Source: CAD feature listing. Evaluate the final solid. Frame: model axes, mm. A direction names the side the tool comes from. Round coordinates to 2 decimals unless told otherwise and drop trailing zeros. Order: outer loops, then holes, each group sorted by start corner. A loop starts at its lowest first (then second) coordinate and runs counter-clockwise, first axis right, second up. Notation, with made-up numbers: (76, 84) -> (113, 84) arc R23 ccw to (113, 99) -> close; hole circle Ø4 at (-27, 69.5). An arc over 180 degrees is marked (long way). Answer as CSV lines item,"result". Start each with the question number.
(1) Contact query for a flat-ended pin moving along its axis: P1, Ø4, axis at x = 2, z = 37, coming from the +Y side. Output: stop coordinate, or through.
(2) Section query B-B (z = 27.5). Output: boundary loops of the cut face in (x, y).
(3) Section query A-A (y = 2.95). Output: boundary loops of the cut face in (x, z), plus the area to 3 significant figures.
(4) Set-up query: faces 1 (the cylindrical face through (-0.2, 0.56, -38.91)), 2 (the flat face through (-0.09, 1.1, 35.77)). Return all of +Z, -Z, +X, -X, +Y, -Y with unobstructed straight access to the full face (end or side cutting, diameter ignored); none if empty.
(5) Pull-direction query (Z, two-part tool) for faces 3 (the flat face through (11.25, 2, 1)), 4 (the cylindrical face through (-0.2, 0.56, -11.26)), 5 (the cylindrical face through (10.537, 2.021, 41.748)); classes: +Z half, -Z half, draft (parallel to the pull), parting line (faces both ways), or undercut.
(6) Section query C-C (x = 0). Count the separate pieces of the cut face and the enclosed holes in it, plus the area to 3 significant figures.
(7) Line query: line 1 along Z through (x, y) = (-3, 3.9); line 2 along X through (y, z) = (3, -7.5); line 3 along Y through (x, z) = (-3.5, 11). Output: solid intervals per line, ascending. Write a range as from..to.
Autodesk Inventor part; units mm, degrees
ref_plane "YZ Plane" through (0, 0, 0) normal (1, 0, 0) x (0, 1, 0)
ref_plane "XZ Plane" through (0, 0, 0) normal (0, 1, 0) x (-1, 0, 0)
ref_plane "XY Plane" through (0, 0, 0) normal (0, 0, 1) x (1, 0, 0)
sketch "Szkic1" plane through (0, 0, 0) normal (0, 1, 0) x (-1, 0, 0)
  line L0 (8.75, 42.5) -> (-8.75, 42.5)
  line L1 (-11.25, 40) -> (-11.25, -40)
  line L2 (-8.75, -42.5) -> (8.75, -42.5)
  line L3 (11.25, -40) -> (11.25, 40)
  line L4 (-11.25, 42.5) -> (11.25, -42.5)
  line L5 (-11.25, -42.5) -> (11.25, 42.5)
  arc A0 (11.25, 40) -> (8.75, 42.5) centre (8.75, 40) ccw
  arc A1 (-8.75, 42.5) -> (-11.25, 40) centre (-8.75, 40) ccw
  arc A2 (-11.25, -40) -> (-8.75, -42.5) centre (-8.75, -40) ccw
  arc A3 (8.75, -42.5) -> (11.25, -40) centre (8.75, -40) ccw
  point P0 (0, 0)
  point P1 (0, 0)
  dimension "d0" = 22.5
  dimension "d1" = 85
  dimension "d2" = 2.5
extrude "Wyciągnięcie proste1" add sketch "Szkic1" along normal blind 4.1
sketch "Szkic2" plane through (0, 4.1, 0) normal (0, 1, 0) x (1, 0, 0)
  line L0 (-6.3, -35) -> (6.3, -35)
  line L1 (6.3, -35) -> (6.3, -12.2)
  line L2 (6.3, -12.2) -> (-6.3, -12.2)
  line L3 (-6.3, -12.2) -> (-6.3, -35)
  line L4 (-8.75, -42.5) -> (8.75, -42.5)
  line L5 (11.25, -40) -> (11.25, 40)
  line L6 (-6.3, 12.2) -> (6.3, 12.2)
  line L7 (6.3, 12.2) -> (6.3, 35)
  line L8 (6.3, 35) -> (-6.3, 35)
  line L9 (-6.3, 35) -> (-6.3, 12.2)
  line L10 (-15.75, 0) -> (15.75, 0)
  point P0 (0, 0)
  point P1 (0, -35)
  dimension "d5" = 12.6
  dimension "d6" = 22.8
  dimension "d7" = 7.5
  dimension "d8" = 11.25
extrude "Wyciągnięcie proste2" cut sketch "Szkic2" against normal blind 4.1
sketch "Szkic4" plane through (0, 4.1, 0) normal (0, 1, 0) x (1, 0, 0)
  line L0 (-6.3, -39.85) -> (6.3, -39.85)
  line L1 (6.3, -39.85) -> (6.3, -7.35)
  line L2 (6.3, -7.35) -> (-6.3, -7.35)
  line L3 (-6.3, -7.35) -> (-6.3, -39.85)
  line L4 (6.3, -35) -> (-6.3, -35)
  line L5 (-6.3, -12.2) -> (6.3, -12.2)
  line L6 (-6.3, 7.35) -> (6.3, 7.35)
  line L7 (6.3, 7.35) -> (6.3, 39.85)
  line L8 (6.3, 39.85) -> (-6.3, 39.85)
  line L9 (-6.3, 39.85) -> (-6.3, 7.35)
  line L10 (6.3, 12.2) -> (-6.3, 12.2)
  line L11 (-6.3, 35) -> (6.3, 35)
  point P0 (0, 0)
  dimension "d11" = 4.85
  dimension "d12" = 4.85
  dimension "d13" = 4.85
  dimension "d14" = 4.85
extrude "Wyciągnięcie proste3" cut sketch "Szkic4" against normal blind 3 contours L3 L4 L1 L0 | L3 L2 L1 L5 | L9 L10 L7 L6 | L9 L8 L7 L11
sketch "Szkic5" plane through (0, 1.1, 0) normal (0, 1, 0) x (1, 0, 0)
  circle A0 centre (0, -37.425) radius 1.5
  circle A1 centre (0, -9.775) radius 1.5
  circle A2 centre (0, 9.775) radius 1.5
  circle A3 centre (0, 37.425) radius 1.5
  line L0 (-6.3, -35) -> (6.3, -35)
  line L1 (6.3, -12.2) -> (-6.3, -12.2)
  line L2 (-6.3, 12.2) -> (6.3, 12.2)
  line L3 (6.3, 35) -> (-6.3, 35)
  point P0 (0, 0)
  point P1 (0, -35)
  point P2 (0, -12.2)
  point P3 (0, 12.2)
  point P4 (0, 35)
  dimension "d17" = 3
  dimension "d18" = 3
  dimension "d19" = 3
  dimension "d20" = 3
  dimension "d21" = 2.425
  dimension "d22" = 2.425
  dimension "d23" = 2.425
  dimension "d24" = 2.425
extrude "Wyciągnięcie proste4" cut sketch "Szkic5" against normal blind 3
properties part number "arm_medium_part"
Answer block:
1,P1,"y = 1.1"
2,outline,"(-11.25, 0) -> (-6.3, 0) -> (-6.3, 4.1) -> (-11.25, 4.1) -> close; (6.3, 0) -> (11.25, 0) -> (11.25, 4.1) -> (6.3, 4.1) -> close"
3,outline,"(-11.25, -40) arc R2.5 ccw to (-8.75, -42.5) -> (8.75, -42.5) arc R2.5 ccw to (11.25, -40) -> (11.25, 40) arc R2.5 ccw to (8.75, 42.5) -> (-8.75, 42.5) arc R2.5 ccw to (-11.25, 40) -> close; hole (-6.3, -39.85) -> (6.3, -39.85) -> (6.3, -7.35) -> (-6.3, -7.35) -> close; hole (-6.3, 7.35) -> (6.3, 7.35) -> (6.3, 39.85) -> (-6.3, 39.85) -> close"
3,area,"1,090 mm2"
4,face 1,"+Y, -Y"
4,face 2,"+Y"
5,face 3,"draft"
5,face 4,"undercut"
5,face 5,"+Z half"
6,separate pieces,"7"
6,enclosed holes,"0"
6,area,"90.1 mm2"
7,line 1,"-42.5..-39.85, -7.35..7.35, 39.85..42.5"
7,line 2,"-11.25..-6.3, 6.3..11.25"
7,line 3,"0..1.1"
